For this review, take the finished solid that the model builds, in its own axes (mm). A direction names the side the tool comes from. Give positions to 0.01 mm unless a question says otherwise; leave off trailing zeros. Loops run counter-clockwise (first coordinate to the right, second up) from the corner with the lowest first, then second, coordinate; pieces in that order, holes last. Notation, with made-up numbers: (-16.5, -36) - (29.5, -36) arc R17 cw to (29.5, -32) - close; hole circle Ø2 at (51, -12.75). An arc over 180 degrees is marked (long way). Answer in a Markdown table with one row per item.
```python
from build123d import *

# Parameters (mm, degrees)
BOSS_EXTRUDE1_DEPTH = 3.175
BOSS_EXTRUDE2_START = -3.175
SKETCH2_R           = 2.24506403
BOSS_EXTRUDE2_DEPTH = 69.85
SKETCH4_R           = 4.7625
BOSS_EXTRUDE4_DEPTH = 19.05
SKETCH5_R           = 4.7625
BOSS_EXTRUDE5_DEPTH = 52.07


with BuildPart() as part:
    # Sketch1 → Boss-Extrude1 (new body)
    with BuildSketch(Plane.XY):
        Polygon((0, 0), (0, 50.8), (-87.988181024, 0), align=None)
        Polygon((-76.13891971, 3.175), (-3.175, 3.175), (-3.175, 45.300738686), align=None, mode=Mode.SUBTRACT)
    extrude(amount=BOSS_EXTRUDE1_DEPTH)

    # Sketch2 → Boss-Extrude2 (add)
    with BuildSketch(Plane(origin=(0, 0, 0), x_dir=(0, 0, -1), z_dir=(1, 0, 0)).offset(BOSS_EXTRUDE2_START)):
        with Locations(Location((-1.5875, 1.5875, 0), (0, 0, 45))):
            Circle(SKETCH2_R)
    extrude(amount=-BOSS_EXTRUDE2_DEPTH)

    # Sketch4 → Boss-Extrude4 (add, symmetric)
    with BuildSketch(Plane(origin=(0, 22.86, 0), x_dir=(-1, 0, 0), z_dir=(0, -1, 0))):
        with Locations(Location((1.5875, -1.5875, 0), (0, 0, 356.177446271))):
            Circle(SKETCH4_R)
    extrude(amount=BOSS_EXTRUDE4_DEPTH, both=True)

    # Sketch5 → Boss-Extrude5 (add, symmetric)
    with BuildSketch(Plane(origin=(-32.995567884, -19.05, 0), x_dir=(0, 0, -1), z_dir=(-0.8660254037844416, -0.49999999999999495, 0))):
        with Locations(Location((-1.5875, -42.406590512, 0), (0, 0, 90))):
            Circle(SKETCH5_R)
    extrude(amount=BOSS_EXTRUDE5_DEPTH, both=True)


solid = part.part
```
1. For faces 1 (the face through (-2, 0, 2)), 2 (the face through (-9.14, 43.77, -0.46)), 3 (the face through (-4, 45, 0)), list the 3-axis set-ups (+Z, -Z, +X, -X, +Y, -Y) from which the entire face can be reached by the end or side of a thin tool; tool diameter is ignored.
Values:
| item | result |
|---|---|
| face 1 | +Z, -Z, +X, -Y |
| face 2 | none |
| face 3 | -Z, +X, +Y |
2. Clearance check with flat-ended pins moving along their axes: pin 1 (0.5 mm diameter, centred on y = 3.5, z = 2.5, fed in from -X); pin 2 (2 mm diameter, centred on x = -21.5, z = -1, fed in from +Y); pin 3 (2.5 mm diameter, centred on x = -3, y = 45, fed in from +Z) (3 decimals); pin 4 (1 mm diameter, centred on x = -39.5, y = 33, fed in from +Z). State where each tip first meets the part, or that it passes through.
Values:
| item | result |
|---|---|
| pin 1 | stops at x = -88.54 |
| pin 2 | stops at y = 42.02 |
| pin 3 | stops at z = 3.175 |
| pin 4 | passes through |
3. Mouldability with a two-part tool opening along X and no side actions: class faces 4 (the face through (-2, 2, 3.175)), 5 (the face through (-1, 41.91, 4)), 6 (the face through (-3.175, 44, 2)), 7 (the face through (0, 2, 2)) as released by +X, released by -X, zero draft, split by the parting line, or undercut.
Values:
| item | result |
|---|---|
| face 4 | zero draft |
| face 5 | undercut |
| face 6 | undercut |
| face 7 | released by +X |
4. We need section B-B, the plane z = -2. Give the boundary of the cut face in (x, y), and give its area (3 significant figures).
Values:
| item | result |
|---|---|
| outline | (-100.86, -5.65) - (-97.73, -11.07) - (-7.54, 41) - (-10.67, 46.42) - close; (-4.72, 3.81) - (1.54, 3.81) - (1.54, 41.91) - (-4.72, 41.91) - close |
| area | 891 mm^2 |
5. We need section A-A, the plane z = 5. Give the boundary of the cut face in (x, y).
Values:
| item | result |
|---|---|
| outline | (-100.95, -5.48) - (-97.63, -11.24) - (-7.44, 40.83) - (-10.77, 46.59) - close; (-4.91, 3.81) - (1.73, 3.81) - (1.73, 41.91) - (-4.91, 41.91) - close |
6. Wall thickness on line 1 (Z direction, x = -63.5, y = 12); line 2 (Y direction, x = -40.5, z = 3); line 3 (X direction, y = -2.5, z = 5.25): over which ranges is each line inside the solid? List them lowest first. Write a range as [from, to].
Values:
| item | result |
|---|---|
| line 1 | z = [-3.17, 6.34] |
| line 2 | y = [-0.16, 3.33], [20.33, 30.84] |
| line 3 | x = [-95.23, -83.05] |
